from build123d import *

# Parameters (mm, degrees)
SKETCH_1_W          = 4
SKETCH_1_H          = 32
SKETCH_1_R          = 0.55
EXTRUDE_1_DEPTH     = 1.6
SKETCH_3_W          = 8.02
SKETCH_3_H          = 6.6
EXTRUDE_2_DEPTH     = 1.6
SKETCH_4_R          = 0.6
CUT_EXTRUDE_1_DEPTH = 1.6
SKETCH_6_W          = 2.01
SKETCH_6_H          = 32
EXTRUDE_3_DEPTH     = 1.6
FILLET_1_R          = 0.5


with BuildPart() as part:
    # 草图1 → 凸台-拉伸1 (new body)
    with BuildSketch(Plane(origin=(0, 0, 0), x_dir=(1, 0, 0), z_dir=(0, 1, 0))):
        Rectangle(SKETCH_1_W, SKETCH_1_H)
        with Locations(Location((0.024094886, 8.850056366, 0), (0, 0, 270))):
            Circle(SKETCH_1_R, mode=Mode.SUBTRACT)
        with Locations(Location((0, 14, 0), (0, 0, 270))):
            Circle(SKETCH_1_R, mode=Mode.SUBTRACT)
        with Locations(Location((0, 3.700112731, 0), (0, 0, 90))):
            Circle(SKETCH_1_R, mode=Mode.SUBTRACT)
    extrude(amount=EXTRUDE_1_DEPTH)

    # 草图3 → 凸台-拉伸2 (add)
    with BuildSketch(Plane(origin=(0, 0, 0), x_dir=(1, 0, 0), z_dir=(0, 1, 0))):
        with Locations((0, -19.3)):
            Rectangle(SKETCH_3_W, SKETCH_3_H)
    extrude(amount=EXTRUDE_2_DEPTH)

    # 草图4 → 切除-拉伸1 (cut)
    with BuildSketch(Plane(origin=(0, 1.6, 0), x_dir=(1, 0, 0), z_dir=(0, 1, 0))):
        with Locations(Location((0, -19.3, 0), (0, 0, 270))):
            Circle(SKETCH_4_R)
        with Locations(Location((-2.54, -19.3, 0), (0, 0, 270))):
            Circle(SKETCH_4_R)
        with Locations(Location((2.54, -19.3, 0), (0, 0, 90))):
            Circle(SKETCH_4_R)
    extrude(amount=-CUT_EXTRUDE_1_DEPTH, mode=Mode.SUBTRACT)

    # 草图6 → 凸台-拉伸3 (add)
    with BuildSketch(Plane(origin=(0, 0, 0), x_dir=(1, 0, 0), z_dir=(0, 1, 0))):
        with Locations((-3.005, 0)):
            Rectangle(SKETCH_6_W, SKETCH_6_H)
    extrude(amount=EXTRUDE_3_DEPTH)

    # 圆角1
    fillet_1_edges = [part.edges().sort_by_distance(p)[0] for p in [
        (4.01, 0.8, 22.6),
        (4.01, 0.8, 16),
        (-4.01, 0.8, 22.6),
        (-4.01, 0.8, -16),
        (2, 0.8, 16),
        (2, 0.8, -16),
    ]]
    fillet(fillet_1_edges, radius=FILLET_1_R)


solid = part.part
Verification items for the finished model (mm, model axes). A direction names the side the tool comes from. Coordinates: 2 decimals unless noted, no trailing zeros. Order: outer loops, then holes, each group sorted by start corner. A loop starts at its lowest first (then second) coordinate and runs counter-clockwise, first axis right, second up. Notation, with made-up numbers: M -15.75,-1.5 L 27.25,-1.5 A12 cw 27.25,3.5 Z; hole C 31.5,-8 d4. An arc over 180 degrees is marked long. Write each question's results on one line, items separated by ' | '.
1) Access from +Z, -Z, +X, -X, +Y, -Y to the whole of each face (thin tool, end or side, straight path). Record for faces 1 (the face through (3, 1, 16)), 2 (the face through (-2.77, 0.811, 19.854)).
Solved:
face 1: -Z, +X, +Y, -Y | face 2: +Y, -Y
2) Section check C-C on z = -14. Record the cut outline in (x, y), plus the area to 3 significant figures.
Solved:
outline: M -4.01,0 L -0.55,0 L -0.55,1.6 L -4.01,1.6 Z; M 0.55,0 L 2,0 L 2,1.6 L 0.55,1.6 Z | area: 7.86 mm²
3) Section check A-A on z = 19.3. Record the cut outline in (x, y).
Solved:
outline: M -4.01,0 L -3.14,0 L -3.14,1.6 L -4.01,1.6 Z; M -1.94,0 L -0.6,0 L -0.6,1.6 L -1.94,1.6 Z; M 0.6,0 L 1.94,0 L 1.94,1.6 L 0.6,1.6 Z; M 3.14,0 L 4.01,0 L 4.01,1.6 L 3.14,1.6 Z
4) Section check D-D on y = 0.5. Record the cut outline in (x, z), plus the area to 3 significant figures.
Solved:
outline: M -4.01,-15.5 A0.5 ccw -3.51,-16 L 1.5,-16 A0.5 ccw 2,-15.5 L 2,15.5 A0.5 cw 2.5,16 L 3.51,16 A0.5 ccw 4.01,16.5 L 4.01,22.1 A0.5 ccw 3.51,22.6 L -3.51,22.6 A0.5 ccw -4.01,22.1 Z; hole C -2.54,19.3 d1.2; hole C 0,19.3 d1.2; hole C 0,-14 d1.1; hole C 0,-3.7 d1.1; hole C 0.02,-8.85 d1.1; hole C 2.54,19.3 d1.2 | area: 239 mm²
5) Section check B-B on x = -2.54. Record the cut outline in (y, z), plus the area to 3 significant figures.
Solved:
outline: M 0,-16 L 1.6,-16 L 1.6,18.7 L 0,18.7 Z; M 0,19.9 L 1.6,19.9 L 1.6,22.6 L 0,22.6 Z | area: 59.8 mm²
6) Scan lines: line 1 along X through (y, z) = (0.5, 19.3); line 2 along Z through (x, y) = (2.5, 0.15); line 3 along X through (y, z) = (1.2, -6). Record each from-to range of solid material in increasing order. Write a range as [from, to].
Solved:
line 1: x = [-4.01, -3.14], [-1.94, -0.6], [0.6, 1.94], [3.14, 4.01] | line 2: z = [16, 18.7], [19.9, 22.6] | line 3: x = [-4.01, 2]
7) Gauge pin test, flat ends, axial feed: pin 1 Ø1.4 at (x, z) = (0.02, -8.85) entering from +Y; pin 2 Ø0.5 at (x, y) = (3, 1) entering from -Z. Record the tip position at first contact, or that the pin passes through.
Solved:
pin 1: stops at y = 1.6 | pin 2: stops at z = 16
8) Release check for a two-part mould opening along X. For faces 3 (the face through (-1, 1, -16)), 4 (the face through (0, 0.8, -9.4)), 5 (the face through (2, 1, 0)), 6 (the face through (-4.01, 1, 4)) record: pulls with the +X half, pulls with the -X half, needs draft (parallel to the pull), parting line crosses it, or undercut.
Solved:
face 3: needs draft | face 4: undercut | face 5: pulls with the +X half | face 6: pulls with the -X half
